CAD build for the part. Positions are in the model's coordinates, mm. A direction names the side the tool comes from. Give positions to 0.01 mm unless a question says otherwise; leave off trailing zeros. Order: outer loops, then holes, each group sorted by start corner. A loop starts at its lowest first (then second) coordinate and runs counter-clockwise, first axis right, second up.
Item 1: Two-plate mould, pull along Y, no slides. Class faces 1 (the flat face through (2.465, 34.27, 2.465)), 2 (the flat face through (5.07, 11.866, 6.098)), 3 (the flat face through (5, 5, -1)), 4 (the flat face through (5.07, 21.88, 6.07)): released by +Y, released by -Y, zero draft, split by the parting line, or undercut.
Item 2: Band-saw the part on D-D on z = -0.5. Give the cut face in (x, y).
Item 3: Which spindle directions (+Z, -Z, +X, -X, +Y, -Y) get a long thin tool onto all of the face, cutting with end or side? Do faces 5 (the flat face through (0, 15, 4)), 6 (the cylindrical face through (2.615, 4.249, -0.493)), 7 (the flat face through (5, 33, 5)), 8 (the flat face through (5.07, 23.134, 6.098)). Say none if no direction does.
Item 4: Wall check: L1, parallel to X at y = 36.5, z = 0.25; L2, parallel to Z at x = 4.25, y = 31; L3, parallel to Z at x = 8.25, y = 9. Give the ranges that are in metal, low to high.
Item 5: Flat gauge pins, fed straight in: P1, Ø4.5, axis at x = 5, y = 34.5, coming from the +Z side; P2, Ø5, axis at x = 1.5, y = 15.5, coming from the -Z side. Where does each tip first touch, or does it go through?
Item 6: Band-saw the part on C-C on y = 10.5. Give the cut face in (x, z).
Item 7: Band-saw the part on A-A on z = 4.25. Give the cut face in (x, y).
Autodesk Inventor part; units mm, degrees
ref_plane "YZ Plane" through (0, 0, 0) normal (1, 0, 0) x (0, 1, 0)
ref_plane "XZ Plane" through (0, 0, 0) normal (0, 1, 0) x (-1, 0, 0)
ref_plane "XY Plane" through (0, 0, 0) normal (0, 0, 1) x (1, 0, 0)
sketch "Esboço1" plane through (0, 0, 0) normal (0, 0, 1) x (1, 0, 0)
  line L0 (0, 0) -> (0, 30)
  line L1 (10, 0) -> (10, 30)
  line L2 (0, 0) -> (10, 0)
  line L3 (0, 30) -> (5, 38.6603)
  line L4 (5, 38.6603) -> (10, 30)
  dimension "d0" = 30
  dimension "d3" = 30
  dimension "d4" = 10
extrude "Extrusão1" add sketch "Esboço1" along normal blind 5
sketch "Esboço3" plane through (10, 0, 0) normal (1, 0, 0) x (0, 0, -1)
  line L0 (-5, 30) -> (-5, 0)
  line L1 (-5, 0) -> (-2.5, 0) construction
  line L2 (-5, 0) -> (-7.1651, 1.25)
  line L3 (-5, 0) -> (-2.5, 0) construction
  line L4 (-7.1651, 1.25) -> (-5, 2.5)
  line L5 (-5, 2.5) -> (-7.1651, 3.75)
  line L6 (-7.1651, 3.75) -> (-5, 5)
  line L7 (-5, 5) -> (-7.1651, 6.25)
  line L8 (-7.1651, 6.25) -> (-5, 7.5)
  line L9 (-5, 7.5) -> (-7.1651, 8.75)
  line L10 (-7.1651, 8.75) -> (-5, 10)
  line L11 (-5, 10) -> (-7.1651, 11.25)
  line L12 (-5, 10) -> (-2.5, 10) construction
  line L13 (-7.1651, 11.25) -> (-5, 12.5)
  line L14 (-5, 12.5) -> (-12.5939, 12.5) construction
  line L15 (-5, 25) -> (-7.1651, 23.75)
  line L16 (-7.1651, 23.75) -> (-5, 22.5)
  line L17 (-5, 22.5) -> (-7.1651, 21.25)
  line L18 (-7.1651, 21.25) -> (-5, 20)
  line L19 (-5, 20) -> (-7.1651, 18.75)
  line L20 (-7.1651, 18.75) -> (-5, 17.5)
  line L21 (-5, 17.5) -> (-7.1651, 16.25)
  line L22 (-7.1651, 16.25) -> (-5, 15)
  line L23 (-5, 15) -> (-7.1651, 13.75)
  line L24 (-7.1651, 13.75) -> (-5, 12.5)
  line L25 (-5, 25) -> (-7.1651, 26.25)
  line L26 (-7.1651, 26.25) -> (-5, 27.5)
  line L27 (-5, 27.5) -> (-7.1651, 28.75)
  line L28 (-7.1651, 28.75) -> (-5, 30)
  line L29 (-5, 30) -> (-5, 38.6603)
  line L30 (-5, 30) -> (-5, 0)
  point P0 (0, 0)
  dimension "d10" = 2.5
  dimension "d11" = 150
  dimension "d12" = 2.5
  dimension "d13" = 2.5
  dimension "d14" = 2.5
  dimension "d15" = 2.5
  dimension "d16" = 150
extrude "Extrusão2" add sketch "Esboço3" against normal blind 10
sketch "Esboço4" plane through (0, 0, 0) normal (0, 0, -1) x (-1, 0, 0)
  circle A0 centre (-5, 5) radius 2.5
  point P0 (0, 0)
  dimension "d19" = 5
extrude "Extrusão3" add sketch "Esboço4" along normal blind 1
properties part number "Prensas coletor"
The answers:
1. face 1: released by +Y
1. face 2: undercut
1. face 3: zero draft
1. face 4: undercut
2. outline: circle Ø5 at (5, 5)
3. face 5: +Z, -Z, -X, +Y, -Y
3. face 6: -Z
3. face 7: +Z, +X, -X, +Y
3. face 8: +Z, +X, -X
4. L1: x = 3.75 to 6.25
4. L2: z = 0 to 5
4. L3: z = 0 to 6.73
5. P1: stops at z = 5
5. P2: stops at z = 0
6. outline: (0, 0) - (10, 0) - (10, 5.87) - (0, 5.87) - close
7. outline: (0, 0) - (10, 0) - (10, 30) - (5, 38.66) - (0, 30) - close
